Answer from the drawing. Dimensions are ordinates in mm from the lowest x, y and z of the part. Give positions to 0.01 mm unless a question says otherwise; leave off trailing zeros. Write each loop counter-clockwise with the first axis right and the second up, starting at its lowest first coordinate (ties: lowest second). Pieces come first, ordered by that corner, then holes. Notation, with made-up numbers: (-8, -13.5) -> (7, -13.5) arc R12 ccw to (7, 6.5) -> close; hole circle Ø8 at (70.5, -32.75). An arc over 180 degrees is marked (long way). Use a Markdown table: item, result. Add a question column.
Q1. Section A-A, the plane z = 18 is taken. Give the vertices of the cut face in (x, y).
Q2. Section B-B, the plane x = 125.5 is taken. Give the vertices of the cut face in (y, z), plus the area to 3 significant figures.
Q3. Consider line 1 (Z direction, x = 36.5, y = 6.5); line 2 (X direction, y = 10.5, z = 21); line 3 (Z direction, x = 39.5, y = 10.75). Determine where each line is inside the solid, lowest interval first.
Q4. Section C-C, the plane y = 10 is taken. Give the vertices of the cut face in (x, z), plus the area to 3 significant figures.
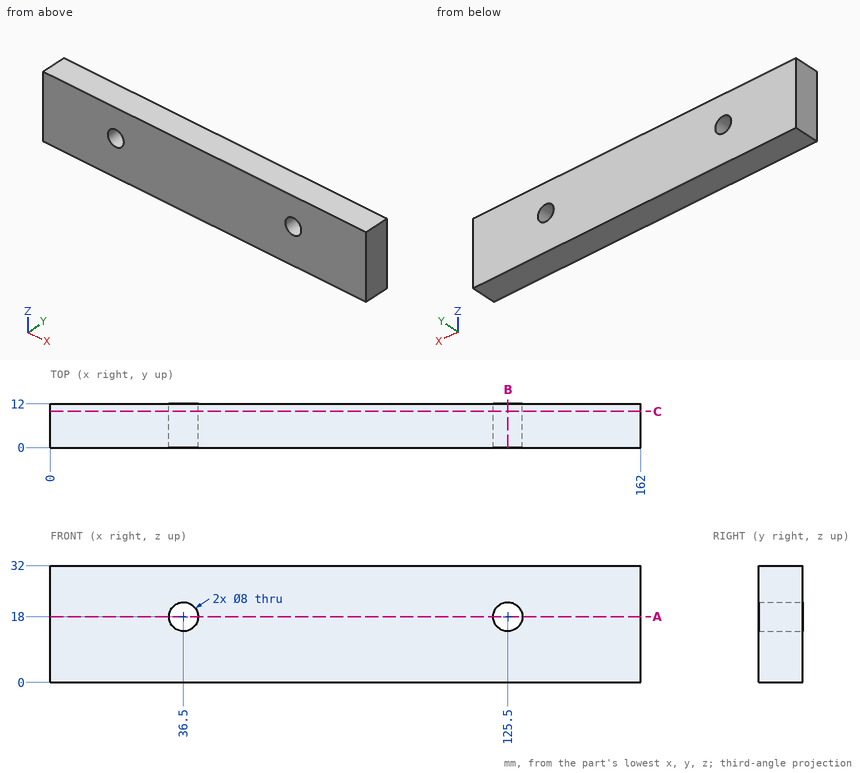
Result set:
| question | item | result |
|---|---|---|
| 1 | outline | (0, 0) -> (32.5, 0) -> (32.5, 12) -> (0, 12) -> close; (40.5, 0) -> (121.5, 0) -> (121.5, 12) -> (40.5, 12) -> close; (129.5, 0) -> (162, 0) -> (162, 12) -> (129.5, 12) -> close |
| 2 | outline | (0, 0) -> (12, 0) -> (12, 14) -> (0, 14) -> close; (0, 22) -> (12, 22) -> (12, 32) -> (0, 32) -> close |
| 2 | area | 288 mm2 |
| 3 | line 1 | z = 0 to 14, 22 to 32 |
| 3 | line 2 | x = 0 to 33.85, 39.15 to 122.85, 128.15 to 162 |
| 3 | line 3 | z = 0 to 15.35, 20.65 to 32 |
| 4 | outline | (0, 0) -> (162, 0) -> (162, 32) -> (0, 32) -> close; hole circle Ø8 at (36.5, 18); hole circle Ø8 at (125.5, 18) |
| 4 | area | 5,080 mm2 |
